Part print with two shaded views. Sizes in mm from the minimum x, y, z corner. A direction names the side the tool comes from. Coordinates: 2 decimals unless noted, no trailing zeros. Write each loop counter-clockwise with the first axis right and the second up, starting at its lowest first coordinate (ties: lowest second). Pieces come first, ordered by that corner, then holes.
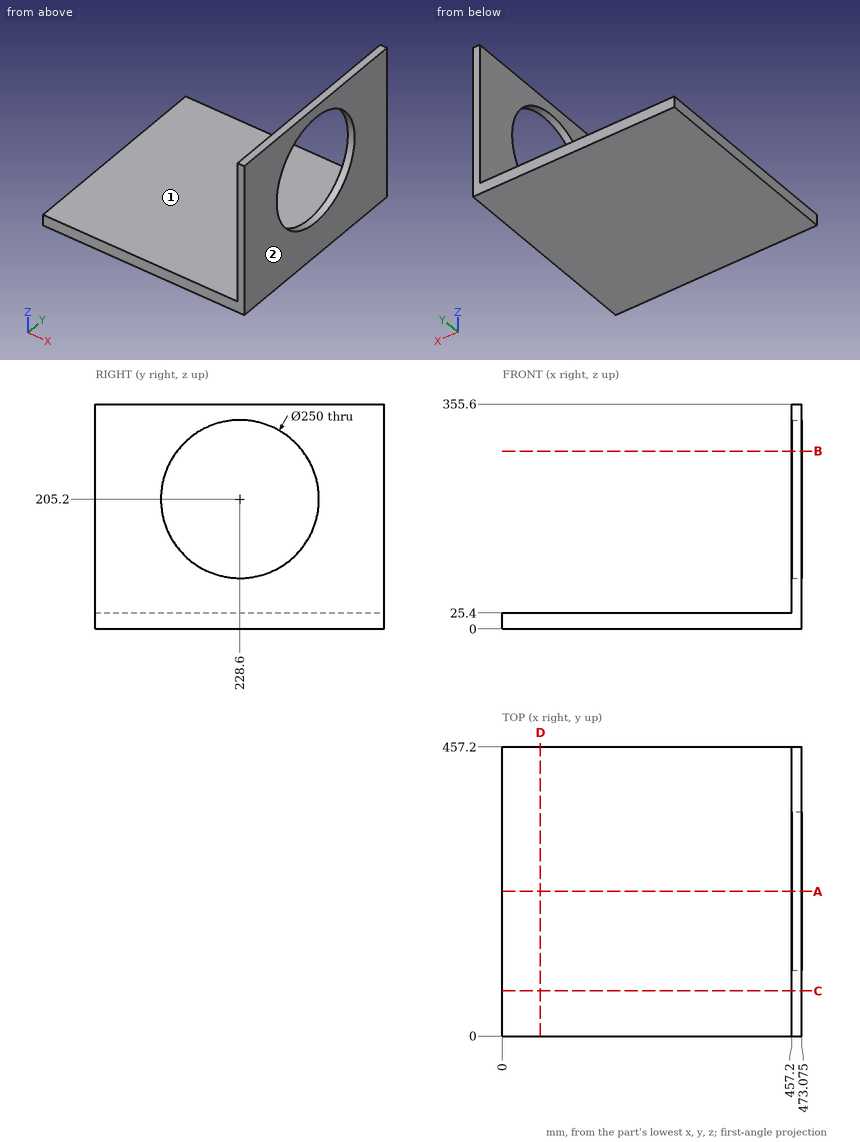
(1) Slice it at C-C, the plane y = 71.5. List the corners of the cut face in (x, z) (1 decimal).
(2) 3-axis set-ups, long thin cutter, end or side, ignore diameter. For the marked faces 1 and 2: which of +Z, -Z, +X, -X, +Y, -Y reach the whole face in a straight line?
(3) Probe L1, parallel to Z at x = 467, y = 228; L2, parallel to Z at x = 93, y = 271.5; L3, parallel to X at y = 86, z = 140.5 (1 decimal). List the from-to ranges inside material, lowest first.
(4) Slice it at A-A, the plane y = 228.6. List the corners of the cut face in (x, z) (1 decimal), and give its area (3 significant figures).
(5) Slice it at B-B, the plane z = 281. List the corners of the cut face in (x, y) (1 decimal).
(6) Flat gauge pins, fed straight in: P1, Ø12, axis at y = 87, z = 38, coming from the -X side; P2, Ø3, axis at x = 195, y = 318.5, coming from the +Z side. Where does each tip first touch, or does it go through?
(7) Slice it at D-D, the plane x = 60. List the corners of the cut face in (y, z).
Results:
1. outline: (0, 0) - (473.1, 0) - (473.1, 355.6) - (457.2, 355.6) - (457.2, 25.4) - (0, 25.4) - close
2. face 1: +Z, -X, +Y, -Y
2. face 2: +Z, -Z, +X, +Y, -Y
3. L1: z = 0 to 80.2, 330.2 to 355.6
3. L2: z = 0 to 25.4
3. L3: x = 457.2 to 473.1
4. outline: (0, 0) - (473.1, 0) - (473.1, 80.2) - (457.2, 80.2) - (457.2, 25.4) - (0, 25.4) - close; (457.2, 330.2) - (473.1, 330.2) - (473.1, 355.6) - (457.2, 355.6) - close
4. area: 13,300 mm2
5. outline: (457.2, 0) - (473.1, 0) - (473.1, 129.2) - (457.2, 129.2) - close; (457.2, 328) - (473.1, 328) - (473.1, 457.2) - (457.2, 457.2) - close
6. P1: stops at x = 457.2
6. P2: stops at z = 25.4
7. outline: (0, 0) - (457.2, 0) - (457.2, 25.4) - (0, 25.4) - close
